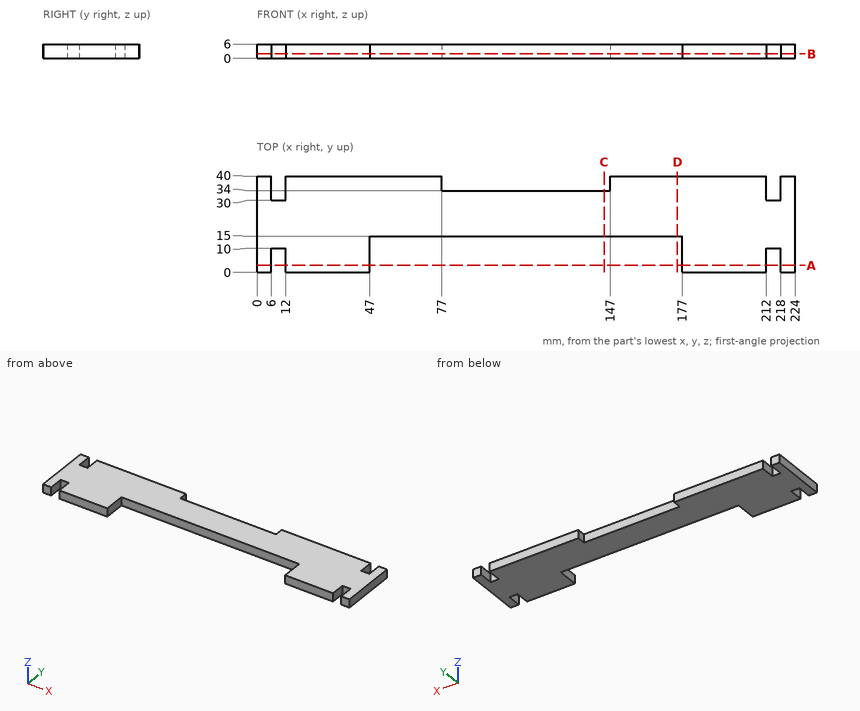
Here's the drawing with two shaded views (mm, measured from the low corner). I have some questions. Coordinates: 2 decimals unless noted, no trailing zeros. Order: outer loops, then holes, each group sorted by start corner. A loop starts at its lowest first (then second) coordinate and runs counter-clockwise, first axis right, second up. Notation, with made-up numbers: (53.25, -11.75) -> (70.25, -11.75) arc R29 cw to (70.25, 9.25) -> close; hole circle Ø4 at (15, 28). An arc over 180 degrees is marked (long way). One line per question, with ' | ' between items.
Q1. If I drill on L1, parallel to X at y = 37.5, z = 5.75; L2, parallel to X at y = 32, z = 1.2; L3, parallel to X at y = 8.5, z = 5.7, over which ranges is the centre line in solid material (lowest first)?
Return value:
L1: 0 to 6, 12 to 77, 147 to 212, 218 to 224 | L2: 0 to 6, 12 to 212, 218 to 224 | L3: 0 to 6, 12 to 47, 177 to 212, 218 to 224
Q2. Imagine slicing it at A-A on y = 3. Please give me the cut outline in (x, z), and give its area (3 significant figures).
Return value:
outline: (0, 0) -> (6, 0) -> (6, 6) -> (0, 6) -> close; (12, 0) -> (47, 0) -> (47, 6) -> (12, 6) -> close; (177, 0) -> (212, 0) -> (212, 6) -> (177, 6) -> close; (218, 0) -> (224, 0) -> (224, 6) -> (218, 6) -> close | area: 492 mm²
Q3. Imagine slicing it at B-B on z = 1.85. Please give me the cut outline in (x, y).
Return value:
outline: (0, 0) -> (6, 0) -> (6, 10) -> (12, 10) -> (12, 0) -> (47, 0) -> (47, 15) -> (177, 15) -> (177, 0) -> (212, 0) -> (212, 10) -> (218, 10) -> (218, 0) -> (224, 0) -> (224, 40) -> (218, 40) -> (218, 30) -> (212, 30) -> (212, 40) -> (147, 40) -> (147, 34) -> (77, 34) -> (77, 40) -> (12, 40) -> (12, 30) -> (6, 30) -> (6, 40) -> (0, 40) -> close
Q4. Imagine slicing it at D-D on x = 175. Please give me the cut outline in (y, z), and give its area (3 significant figures).
Return value:
outline: (15, 0) -> (40, 0) -> (40, 6) -> (15, 6) -> close | area: 150 mm²
Q5. I'm going to push flat-ended pins straight in: P1, Ø3, axis at x = 140.5, z = 2, coming from the +Y side; P2, Ø3, axis at x = 8, z = 2.5, coming from the -Y side; P3, Ø3, axis at x = 115, z = 3, coming from the -Y side. Where does each tip first touch, or does it pass through?
Return value:
P1: y = 34 | P2: y = 10 | P3: y = 15
Q6. Imagine slicing it at C-C on x = 144.5. Please give me the cut outline in (y, z).
Return value:
outline: (15, 0) -> (34, 0) -> (34, 6) -> (15, 6) -> close
